CAD build for the part. Positions are in the model's coordinates, mm. A direction names the side the tool comes from. Give positions to 0.01 mm unless a question says otherwise; leave off trailing zeros. Order: outer loops, then holes, each group sorted by start corner. A loop starts at its lowest first (then second) coordinate and runs counter-clockwise, first axis right, second up.
Item 1: Band-saw the part on A-A on z = 17.75. Count the separate pieces of the cut face and the enclosed holes in it, plus the area to 3 significant figures.
Item 2: Flat gauge pins, fed straight in: P1, Ø2.5, axis at x = 21.78, y = -25.53, coming from the -Z side; P2, Ø4, axis at x = 11.5, y = -14, coming from the +Z side; P3, Ø9, axis at x = 23, y = -27, coming from the -Z side (3 decimals); P4, Ø4, axis at x = 7.5, y = -23, coming from the +Z side (3 decimals). Where does each tip first touch, or does it go through?
Item 3: Band-saw the part on D-D on z = 4.25. Give the cut face in (x, y), plus the area to 3 significant figures.
Item 4: Wall check: L1, parallel to X at y = -13, z = 19.75; L2, parallel to Z at x = 18, y = -21.5 (3 decimals); L3, parallel to X at y = -22, z = 17.75 (3 decimals). Give the ranges that are in metal, low to high.
Item 5: Band-saw the part on B-B on x = 3.5. Give the cut face in (y, z).
Item 6: Two-plate mould, pull along X, no slides. Class faces 1 (the flat face through (9, -30, 7)), 2 (the flat face through (31.3, -9, 13)), 3 (the flat face through (25.775, -25, 7)): released by +X, released by -X, zero draft, split by the parting line, or undercut.
Item 7: Which spindle directions (+Z, -Z, +X, -X, +Y, -Y) get a long thin tool onto all of the face, cutting with end or side? Do faces 4 (the flat face through (13, 1, 22.15)), 5 (the flat face through (16, -4, 1)), 6 (the flat face through (16, -12, 2)). Say none if no direction does.
Item 8: Band-saw the part on C-C on y = -17. Give the cut face in (x, z) (3 decimals), plus the area to 3 significant figures.
Autodesk Inventor part; units mm, degrees
ref_plane "YZ Plane" through (0, 0, 0) normal (1, 0, 0) x (0, 1, 0)
ref_plane "XZ Plane" through (0, 0, 0) normal (0, 1, 0) x (-1, 0, 0)
ref_plane "XY Plane" through (0, 0, 0) normal (0, 0, 1) x (1, 0, 0)
sketch "Sketch1" plane through (0, 0, 0) normal (0, 0, 1) x (1, 0, 0)
  line L0 (0, -2) -> (30.8, -2)
  line L1 (4.3, -2) -> (4.3, -1.5)
  line L2 (30.8, -2) -> (30.8, -4)
  line L3 (30.8, -4) -> (0, -4)
  line L4 (0, -4) -> (0, -2)
  line L5 (2.65, -20) -> (28.15, -20)
  line L6 (2.65, -20) -> (2.65, -4)
  line L7 (28.15, -20) -> (28.15, -4)
  arc A0 (10.3, 4.5) -> (4.3, -1.5) centre (10.3, -1.5) ccw
  line L8 (10.3, 4.5) -> (26.5, -1.5)
  line L9 (26.5, -1.5) -> (26.5, -2)
  line L10 (-1, -14) -> (2.65, -20)
  line L11 (-1, -14) -> (-1, -4)
  line L12 (-0.5, -4) -> (-0.5, -13.8599)
  line L13 (-0.5, -13.8599) -> (2.65, -19.0379)
  line L14 (-1, -4) -> (-0.5, -4)
  line L15 (31.8, -14) -> (28.15, -20)
  line L16 (31.8, -14) -> (31.8, -4)
  line L17 (31.3, -4) -> (31.3, -13.8599)
  line L18 (31.3, -13.8599) -> (28.15, -19.0379)
  line L19 (31.8, -4) -> (31.3, -4)
  point P0 (4.3, 4.5)
  dimension "d0" = 30.8
  dimension "d2" = 6.5
  dimension "d4" = 2
  dimension "d6" = 4.3
  dimension "d9" = 25.5
  dimension "d10" = 16
  dimension "d11" = 6
  dimension "d12" = 0.5
  dimension "d13" = 6
  dimension "d16" = 6
  dimension "d17" = 10
  dimension "d19" = 0.5
extrude "Extrusion1" add sketch "Sketch1" along normal blind 25.5 contours L0 L2 L3 L4
extrude "Extrusion2" add sketch "Sketch1" along normal blind 22.15 contours L1 A0 L8 L9 L0
sketch "Sketch2" plane through (30.8, -4, 0) normal (1, 0, 0) x (0, 0, -1)
  line L0 (-3.35, 8.5) -> (-3.35, 2)
  line L1 (0, 8.5) -> (-22.15, 8.5)
  line L2 (-3.35, 8.5) -> (0, 8.5)
  line L3 (0, 0) -> (-25.5, 0)
  line L4 (0, 2) -> (-22.15, 2)
  line L5 (-3.35, 2) -> (0, 2)
  line L6 (0, 2) -> (0, 8.5)
  point P0 (0, 4)
extrude "Extrusion3" cut sketch "Sketch2" against normal blind 30
extrude "Extrusion4" add sketch "Sketch1" along normal blind 23.5 contours L3 L7 L5 L6 | L6 L10 L11 L14 L12 L13 | L18 L17 L19 L16 L15 L7
sketch "Sketch3" plane through (31.8, -14, 0) normal (1, 0, 0) x (0, 0, -1)
  line L0 (0, 10) -> (-25.5, 10)
  line L1 (0, 10) -> (-2, 10)
  line L2 (-2, 10) -> (-2, -9.6179)
  line L3 (-2, -9.6179) -> (0, -9.6179)
  line L4 (0, -5.0379) -> (0, 10)
  line L5 (0, -9.6179) -> (0, 10)
  line L6 (0, 10) -> (0, -9.6179)
  point P0 (0, 14)
  dimension "d29" = 2
extrude "Extrusion5" cut sketch "Sketch3" against normal blind 40
sketch "Sketch4" plane through (2.65, -20, 23.5) normal (0, -1, 0) x (1, 0, 0)
  line L0 (25.5, -21.5) -> (25.5, 0)
  line L1 (25.5, -21.5) -> (0, 0)
  line L2 (12.75, -10.75) -> (12.75, -21.5)
  line L3 (0, -21.5) -> (25.5, -21.5)
  line L4 (12.75, -21.5) -> (25.5, -21.5)
  line L5 (19.125, -21.5) -> (19.125, 0)
  line L6 (0, 0) -> (25.5, 0)
  line L7 (19.125, -16.125) -> (15.125, -16.125)
  line L8 (15.125, -16.125) -> (15.125, -18.125)
  line L9 (15.125, -18.125) -> (23.125, -18.125)
  line L10 (23.125, -18.125) -> (23.125, -14.125)
  line L11 (23.125, -14.125) -> (15.125, -14.125)
  line L12 (15.125, -14.125) -> (15.125, -16.125)
  line L13 (12.75, -10.75) -> (9.9991, -10.75)
  line L14 (10.375, -16.125) -> (10.375, -18.125)
  line L15 (10.375, -18.125) -> (2.375, -18.125)
  line L16 (2.375, -18.125) -> (2.375, -14.125)
  line L17 (2.375, -14.125) -> (10.375, -14.125)
  line L18 (10.375, -14.125) -> (10.375, -16.125)
  line L19 (15.125, -5.375) -> (15.125, -3.375)
  line L20 (15.125, -3.375) -> (23.125, -3.375)
  line L21 (23.125, -3.375) -> (23.125, -7.375)
  line L22 (23.125, -7.375) -> (15.125, -7.375)
  line L23 (15.125, -7.375) -> (15.125, -5.375)
  line L24 (10.375, -5.375) -> (10.375, -3.375)
  line L25 (10.375, -3.375) -> (2.375, -3.375)
  line L26 (2.375, -3.375) -> (2.375, -7.375)
  line L27 (2.375, -7.375) -> (10.375, -7.375)
  line L28 (10.375, -7.375) -> (10.375, -5.375)
  line L29 (19.125, -14.125) -> (16.7529, -14.125)
  line L30 (19.125, -7.375) -> (15.125, -7.375)
  line L31 (15.125, -3.375) -> (15.125, -7.375)
  line L32 (19.125, -3.375) -> (15.125, -3.375)
  point P0 (-2.65, -23.5)
  dimension "d32" = 4
  dimension "d33" = 2
  dimension "d34" = 8
  dimension "d35" = 4
extrude "Extrusion6" add sketch "Sketch4" along normal blind 10 contours L9 L5 L1 | L1 L5 L11 L10 L9 | L7 L12 L11 L1 | L1 L11 L5 | L5 L9 L8 L7 | L20 L21 L22 L5 | L5 L22 L23 L19 L20 | L25 L24 L28 L27 L1 | L1 L27 L26 L25 | L14 L15 L16 L17 L18
sketch "Sketch5" plane through (25.775, -20, 5.375) normal (0, 0, -1) x (-1, 0, 0)
  circle A0 centre (4, -5.5341) radius 2
  line L0 (23.125, 0) -> (-2.375, 0)
  line L1 (10.375, 0) -> (10.375, -1.7461)
  circle A1 centre (16.75, -5.5341) radius 2
  dimension "d38" = 4
extrude "Extrusion7" cut sketch "Sketch5" against normal blind 40
sketch "Sketch6" plane through (10.3, 4.5, 22.15) normal (0.3473, 0.9377, 0) x (0.9377, -0.3473, 0)
  line L0 (17.2754, 18.8) -> (17.2754, 0)
  line L1 (17.2754, 9.4) -> (-10.0504, 9.4)
  line L2 (17.4491, 0) -> (-3.3689, 0)
  line L3 (7.0401, 0) -> (7.0357, 14.775)
  line L4 (7.0357, 12.775) -> (7.0357, 16.775)
  line L5 (7.0373, 9.4) -> (17.4491, 0)
  circle A0 centre (12.2432, 9.4) radius 2.75
  line L6 (7.0401, 0) -> (0, 9.4)
  line L7 (0, 18.8) -> (0, 0)
  line L8 (7.0373, 9.4) -> (7.0375, 8.65)
  line L9 (7.0375, 8.65) -> (1.0375, 8.6482)
  line L10 (1.0375, 8.6482) -> (1.0371, 10.1482)
  line L11 (1.0371, 10.1482) -> (7.0371, 10.15)
  line L12 (7.0373, 9.4) -> (7.0371, 10.15)
  line L13 (1.0371, 10.1482) -> (7.0371, 10.15)
  circle A1 centre (12.2432, 9.4) radius 3.35
  line L14 (1.4371, 10.1484) -> (1.4374, 9.0484)
  line L15 (1.4374, 9.0484) -> (6.6374, 9.0499)
  line L16 (6.6374, 9.0499) -> (6.6373, 9.3999)
  line L17 (1.0372, 9.7482) -> (7.0372, 9.75)
  line L18 (6.6373, 9.3999) -> (6.6371, 10.1499)
  point P0 (-8.0959, 22.15)
  point P1 (1.4372, 9.7484)
  point P2 (6.6372, 9.7499)
  dimension "d41" = 5.5
  dimension "d42" = 0.75
  dimension "d43" = 6
  dimension "d44" = 1.5
  dimension "d45" = 0.6
  dimension "d46" = 0.4
  dimension "d47" = 0.4
  dimension "d48" = 0.4
extrude "Extrusion8" add sketch "Sketch6" along normal blind 0.01 contours A1 L1 A0 | L1 A0 A1 | L3 L9 L10 L1 L14 L15 L16 | L1 L18 L17 L3 | L17 L18 L11 L3 | L1 L10 L17 L14 | L17 L14 L11 L18 | L17 L10 L11 L14
sketch "Sketch7" plane through (13.025, -20, 5.375) normal (0, 0, -1) x (-1, 0, 0)
  circle A0 centre (4, -5.5341) radius 2
properties part number "Tecla On_Off - Máquina - DMI"
The answers:
1. separate pieces: 1
1. enclosed holes: 2
1. area: 709 mm2
2. P1: passes through
2. P2: stops at z = 23.5
2. P3: stops at z = 5.375
2. P4: stops at z = 20.125
3. outline: (-1, -14) - (2.65, -20) - (28.15, -20) - (31.8, -14) - (31.8, -4) - (31.3, -4) - (31.3, -13.86) - (28.15, -19.04) - (28.15, -4) - (30.8, -4) - (30.8, -2) - (26.5, -2) - (26.5, -1.5) - (10.3, 4.5) arc R6 ccw to (4.3, -1.5) - (4.3, -2) - (0, -2) - (0, -4) - (2.65, -4) - (2.65, -19.04) - (-0.5, -13.86) - (-0.5, -4) - (-1, -4) - close
3. area: 574 mm2
4. L1: x = -1 to -0.5, 2.65 to 28.15, 31.3 to 31.8
4. L2: z = 5.375 to 9.375, 16.125 to 20.125
4. L3: x = 5.025 to 13.025, 17.775 to 25.775
5. outline: (-20, 2) - (-4, 2) - (-4, 0) - (-2, 0) - (-2, 25.5) - (-4, 25.5) - (-4, 23.5) - (-20, 23.5) - close
6. face 1: zero draft
6. face 2: undercut
6. face 3: released by +X
7. face 4: +Z, +X, -X, +Y
7. face 5: none
7. face 6: -Z, +X, -X, -Y
8. outline: (0.825, 2) - (1.41, 2) - (1.41, 23.5) - (0.825, 23.5) - close; (2.65, 2) - (28.15, 2) - (28.15, 23.5) - (2.65, 23.5) - close; (29.39, 2) - (29.975, 2) - (29.975, 23.5) - (29.39, 23.5) - close
8. area: 573 mm2
